from build123d import *

# Parameters (mm, degrees)
F0_W     = 304.8
F0_H     = 152.4
F1_DEPTH = 4.4958
F2_R     = 5.08
F3_R     = 4.8895
F4_DEPTH = 4.4968


with BuildPart() as f1:
    # F0 (on Top) → F1 (new body)
    with BuildSketch(Plane.XY):
        Rectangle(F0_W, F0_H)
    extrude(amount=F1_DEPTH)

    # F2
    f2_edges = [f1.edges().sort_by_distance(p)[0] for p in [
        (-152.4, 76.2, 2.2479),
        (-152.4, -76.2, 2.2479),
        (152.4, -76.2, 2.2479),
        (152.4, 76.2, 2.2479),
    ]]
    fillet(f2_edges, radius=F2_R)

    # F3 (on face) → F4 (cut, through all)
    with BuildSketch(Plane.XY.offset(4.4958)):
        with Locations((-144.3355, 68.1355)):
            Circle(F3_R)
        with Locations((144.3355, 68.1355)):
            Circle(F3_R)
        with Locations((144.3355, -68.1355)):
            Circle(F3_R)
        with Locations((-144.3355, -68.1355)):
            Circle(F3_R)
    extrude(amount=-F4_DEPTH, mode=Mode.SUBTRACT)


solid = f1.part
Verification items for the finished model (mm, model axes). Give positions to 0.01 mm unless a question says otherwise; leave off trailing zeros. Answer as CSV lines item,"result".
Q1. Release check for a two-part mould opening along Y. For faces 1 (the cylindrical face through (-148.216, -71.111, 2.279)), 2 (the flat face through (-2, 1, 0)), 3 (the cylindrical face through (149, 69.6, 2.3)) record: +Y half, -Y half, draft (parallel to the pull), parting line (faces both ways), or undercut.
Solutions:
face 1,"undercut"
face 2,"draft"
face 3,"undercut"
Q2. Scan line: probe 1 along X at (y, z) = (65.5, 1.35). Record every from-to range of solid material in increasing order.
Solutions:
probe 1,"x = -152.4 to -148.45, -140.22 to 140.22, 148.45 to 152.4"
Q3. Depth check by flat-ended pin: pin 1 (3 mm diameter, centred on x = -71, y = 38.5, fed in from -Z). Enter the tip coordinate at first touch or a pass-through.
Solutions:
pin 1,"stops at z = 0"
